Here's how the part is built. I have some questions about the finished solid (model axes, mm). Face numbers are marked on the shaded views. A direction names the side the tool comes from. Round coordinates to 2 decimals unless told otherwise and drop trailing zeros. Order: outer loops, then holes, each group sorted by start corner. A loop starts at its lowest first (then second) coordinate and runs counter-clockwise, first axis right, second up. Notation, with made-up numbers: (-26, -18) - (-13, -18) arc R13 cw to (-13, -10) - close; hole circle Ø7 at (-12, -30). An arc over 180 degrees is marked (long way). Answer as a JSON object with one key per item and string values.
```python
from build123d import *

# Parameters (mm, degrees)
SKETCH1_R               = 1.5
SKETCH1_R_2             = 3
SKETCH1_R_3             = 2
SKETCH1_W               = 12.75
SKETCH1_H               = 8.25
BOSS_EXTRUDE1_DEPTH     = 6.35
FILLET1_R               = 1.5
SKETCH3_W               = 129.678218063
SKETCH3_H               = 13.276015012
CUT_EXTRUDE1_DEPTH      = 56
SKETCH4_W               = 14.25
SKETCH4_H               = 6.35
SKETCH4_W_2             = 20.25
SKETCH4_W_3             = 16.5
BOSS_EXTRUDE2_DEPTH     = 25
SKETCH5_W               = 158.83803675
SKETCH5_H               = 69.224935419
CUT_EXTRUDE2_DEPTH      = 86
CUT_EXTRUDE3_DEPTH      = 10
CUT_EXTRUDE3_DEPTH_BACK = 49
SKETCH6_W               = 0.1
SKETCH6_H               = 6.35
SKETCH7_W               = 88.464513538
SKETCH7_H               = 23.115624737
CUT_EXTRUDE4_DEPTH      = 84


with BuildPart() as part:
    # Sketch1 → Boss-Extrude1 (new body)
    with BuildSketch(Plane(origin=(0, 0, 0), x_dir=(1, 0, 0), z_dir=(0, 1, 0))):
        Polygon((0, 20), (0, 104), (12, 104), (14, 93), (26, 93), (26, 107), (33.5, 114), (62.5, 114), (70, 107), (70, 93), (82, 93), (84, 104), (96, 104), (96, 20), (89, 9), (89, 0), (62, 0), (62, 8), (34, 8), (34, 0), (7, 0), (7, 9), align=None)
        with Locations(Location((12.5, 3, 0), (0, 0, 270))):
            Circle(SKETCH1_R, mode=Mode.SUBTRACT)
        with Locations(Location((28, 3, 0), (0, 0, 270))):
            Circle(SKETCH1_R, mode=Mode.SUBTRACT)
        with Locations(Location((68, 3, 0), (0, 0, 90))):
            Circle(SKETCH1_R, mode=Mode.SUBTRACT)
        with Locations(Location((83.5, 3, 0), (0, 0, 90))):
            Circle(SKETCH1_R, mode=Mode.SUBTRACT)
        with Locations(Location((14, 13, 0), (0, 0, 270))):
            Circle(SKETCH1_R_2, mode=Mode.SUBTRACT)
        with Locations(Location((27, 13, 0), (0, 0, 270))):
            Circle(SKETCH1_R_2, mode=Mode.SUBTRACT)
        with Locations(Location((69, 13, 0), (0, 0, 90))):
            Circle(SKETCH1_R_2, mode=Mode.SUBTRACT)
        with Locations(Location((82, 13, 0), (0, 0, 90))):
            Circle(SKETCH1_R_2, mode=Mode.SUBTRACT)
        with Locations(Location((22.75, 42.455027657, 0), (0, 0, 270))):
            Circle(SKETCH1_R, mode=Mode.SUBTRACT)
        with Locations(Location((22.75, 51.751081058, 0), (0, 0, 270))):
            Circle(SKETCH1_R, mode=Mode.SUBTRACT)
        with Locations(Location((73.25, 42.455027657, 0), (0, 0, 90))):
            Circle(SKETCH1_R, mode=Mode.SUBTRACT)
        with Locations(Location((73.25, 51.751081058, 0), (0, 0, 90))):
            Circle(SKETCH1_R, mode=Mode.SUBTRACT)
        with Locations(Location((18, 72.75, 0), (0, 0, 270))):
            Circle(SKETCH1_R, mode=Mode.SUBTRACT)
        with Locations(Location((28, 65.75, 0), (0, 0, 270))):
            Circle(SKETCH1_R, mode=Mode.SUBTRACT)
        with Locations(Location((68, 65.75, 0), (0, 0, 90))):
            Circle(SKETCH1_R, mode=Mode.SUBTRACT)
        with Locations(Location((78, 72.75, 0), (0, 0, 90))):
            Circle(SKETCH1_R, mode=Mode.SUBTRACT)
        with Locations(Location((36.5, 76.75, 0), (0, 0, 270))):
            Circle(SKETCH1_R_3, mode=Mode.SUBTRACT)
        with Locations(Location((59.5, 76.75, 0), (0, 0, 90))):
            Circle(SKETCH1_R_3, mode=Mode.SUBTRACT)
        with Locations(Location((35.5, 89, 0), (0, 0, 270))):
            Circle(SKETCH1_R, mode=Mode.SUBTRACT)
        with Locations(Location((35.5, 106.5, 0), (0, 0, 270))):
            Circle(SKETCH1_R, mode=Mode.SUBTRACT)
        with Locations(Location((60.5, 89, 0), (0, 0, 90))):
            Circle(SKETCH1_R, mode=Mode.SUBTRACT)
        with Locations(Location((60.5, 106.5, 0), (0, 0, 90))):
            Circle(SKETCH1_R, mode=Mode.SUBTRACT)
        with Locations(Location((44, 26, 0), (0, 0, 270))):
            Circle(SKETCH1_R, mode=Mode.SUBTRACT)
        with Locations(Location((52, 26, 0), (0, 0, 90))):
            Circle(SKETCH1_R, mode=Mode.SUBTRACT)
        with Locations(Location((52, 74, 0), (0, 0, 270))):
            Circle(SKETCH1_R, mode=Mode.SUBTRACT)
        with Locations(Location((44, 74, 0), (0, 0, 90))):
            Circle(SKETCH1_R, mode=Mode.SUBTRACT)
        with Locations(Location((48, 97.75, 0), (0, 0, 270))):
            Circle(SKETCH1_R_3, mode=Mode.SUBTRACT)
        with Locations((69.875, 25.875)):
            Rectangle(SKETCH1_W, SKETCH1_H, mode=Mode.SUBTRACT)
        with Locations((26.125, 25.875)):
            Rectangle(SKETCH1_W, SKETCH1_H, mode=Mode.SUBTRACT)
        with Locations((69.875, 81.875)):
            Rectangle(SKETCH1_W, SKETCH1_H, mode=Mode.SUBTRACT)
        with Locations((26.125, 81.875)):
            Rectangle(SKETCH1_W, SKETCH1_H, mode=Mode.SUBTRACT)
        with BuildLine():
            Line((3, 75), (7, 75))
            ThreePointArc((7, 75), (9, 73), (7, 71))
            Line((7, 71), (3, 71))
            ThreePointArc((3, 71), (1, 73), (3, 75))
        make_face(mode=Mode.SUBTRACT)
        with BuildLine():
            Line((93, 75), (89, 75))
            ThreePointArc((89, 75), (87, 73), (89, 71))
            Line((89, 71), (93, 71))
            ThreePointArc((93, 71), (95, 73), (93, 75))
        make_face(mode=Mode.SUBTRACT)
        with BuildLine():
            Line((93, 37), (89, 37))
            ThreePointArc((89, 37), (87, 35), (89, 33))
            Line((89, 33), (93, 33))
            ThreePointArc((93, 33), (95, 35), (93, 37))
        make_face(mode=Mode.SUBTRACT)
        with BuildLine():
            Line((3, 33), (7, 33))
            ThreePointArc((7, 33), (9, 35), (7, 37))
            Line((7, 37), (3, 37))
            ThreePointArc((3, 37), (1, 35), (3, 33))
        make_face(mode=Mode.SUBTRACT)
        with BuildLine():
            Line((15, 48.525154469), (23, 48.525154469))
            ThreePointArc((23, 48.525154469), (24.5, 47.025154469), (23, 45.525154469))
            Line((23, 45.525154469), (15, 45.525154469))
            ThreePointArc((15, 45.525154469), (13.5, 47.025154469), (15, 48.525154469))
        make_face(mode=Mode.SUBTRACT)
        with BuildLine():
            Line((81, 48.525154469), (73, 48.525154469))
            ThreePointArc((73, 48.525154469), (71.5, 47.025154469), (73, 45.525154469))
            Line((73, 45.525154469), (81, 45.525154469))
            ThreePointArc((81, 45.525154469), (82.5, 47.025154469), (81, 48.525154469))
        make_face(mode=Mode.SUBTRACT)
        with BuildLine():
            Line((16.5, 67.75), (16.5, 57.75))
            ThreePointArc((16.5, 57.75), (18, 56.25), (19.5, 57.75))
            Line((19.5, 57.75), (19.5, 67.75))
            ThreePointArc((19.5, 67.75), (18, 69.25), (16.5, 67.75))
        make_face(mode=Mode.SUBTRACT)
        with BuildLine():
            Line((76.5, 67.75), (76.5, 57.75))
            ThreePointArc((76.5, 57.75), (78, 56.25), (79.5, 57.75))
            Line((79.5, 57.75), (79.5, 67.75))
            ThreePointArc((79.5, 67.75), (78, 69.25), (76.5, 67.75))
        make_face(mode=Mode.SUBTRACT)
        with BuildLine():
            Line((46.5, 29), (38, 29))
            Line((38, 29), (38, 71))
            Line((38, 71), (46.5, 71))
            Line((46.5, 71), (46.5, 74))
            ThreePointArc((46.5, 74), (48, 75.5), (49.5, 74))
            Line((49.5, 74), (49.5, 71))
            Line((49.5, 71), (58, 71))
            Line((58, 71), (58, 29))
            Line((58, 29), (49.5, 29))
            Line((49.5, 29), (49.5, 26))
            ThreePointArc((49.5, 26), (48, 24.5), (46.5, 26))
            Line((46.5, 26), (46.5, 29))
        make_face(mode=Mode.SUBTRACT)
    extrude(amount=BOSS_EXTRUDE1_DEPTH)

    # Fillet1
    fillet1_edges = [part.edges().sort_by_distance(p)[0] for p in [
        (19.75, 3.175, -30),
        (19.75, 3.175, -21.75),
        (32.5, 3.175, -21.75),
        (32.5, 3.175, -30),
        (63.5, 3.175, -77.75),
        (76.25, 3.175, -77.75),
        (76.25, 3.175, -86),
        (63.5, 3.175, -86),
        (19.75, 3.175, -86),
        (19.75, 3.175, -77.75),
        (32.5, 3.175, -77.75),
        (32.5, 3.175, -86),
        (58, 3.175, -29),
        (58, 3.175, -71),
        (38, 3.175, -71),
        (38, 3.175, -29),
        (62, 3.175, -8),
        (34, 3.175, -8),
        (34, 3.175, 0),
        (7, 3.175, 0),
        (7, 3.175, -9),
        (0, 3.175, -20),
        (0, 3.175, -104),
        (12, 3.175, -104),
        (14, 3.175, -93),
        (26, 3.175, -93),
        (26, 3.175, -107),
        (33.5, 3.175, -114),
        (62.5, 3.175, -114),
        (70, 3.175, -107),
        (70, 3.175, -93),
        (82, 3.175, -93),
        (84, 3.175, -104),
        (96, 3.175, -104),
        (96, 3.175, -20),
        (89, 3.175, -9),
        (89, 3.175, 0),
        (62, 3.175, 0),
        (76.25, 3.175, -21.75),
        (76.25, 3.175, -30),
        (63.5, 3.175, -30),
        (63.5, 3.175, -21.75),
    ]]
    fillet(fillet1_edges, radius=FILLET1_R)

    # Sketch3 → Cut-Extrude1 (cut)
    with BuildSketch(Plane(origin=(48, 0, 0), x_dir=(0, 0, -1), z_dir=(1, 0, 0))):
        with Locations((58.42243018, 0.940732076)):
            Rectangle(SKETCH3_W, SKETCH3_H)
    extrude(amount=CUT_EXTRUDE1_DEPTH, mode=Mode.SUBTRACT)

    # Sketch4 → Boss-Extrude2 (add)
    with BuildSketch(Plane(origin=(48, 0, 0), x_dir=(0, 0, -1), z_dir=(1, 0, 0))):
        with Locations((106.875, 3.175)):
            Rectangle(SKETCH4_W, SKETCH4_H)
        with Locations((85.625, 3.175)):
            Rectangle(SKETCH4_W_2, SKETCH4_H)
        with Locations((16.25, 3.175)):
            Rectangle(SKETCH4_W_3, SKETCH4_H)
    extrude(amount=BOSS_EXTRUDE2_DEPTH)

    # Mirror1: part across plane


with BuildPart() as part_1:
    add(part.part)
    add(part.part.mirror(Plane(origin=(73, 0, 0), x_dir=(0, 0, 1), z_dir=(1, 0, 0))))

    # Sketch5 → Cut-Extrude2 (cut)
    with BuildSketch(Plane(origin=(75, 0, 0), x_dir=(0, 0, -1), z_dir=(1, 0, 0))):
        with Locations((54.73207584, 3.767679241)):
            Rectangle(SKETCH5_W, SKETCH5_H)
    extrude(amount=CUT_EXTRUDE2_DEPTH, mode=Mode.SUBTRACT)

    # Sketch6 → Cut-Extrude3 (cut, two sides: drawn at the far end of the back side and taken through both)
    with BuildSketch(Plane(origin=(38, 0, 0), x_dir=(0, 0, -1), z_dir=(1, 0, 0)).offset(-CUT_EXTRUDE3_DEPTH_BACK)):
        with Locations((48.95, 3.175)):
            Rectangle(SKETCH6_W, SKETCH6_H)
    extrude(amount=CUT_EXTRUDE3_DEPTH + CUT_EXTRUDE3_DEPTH_BACK, mode=Mode.SUBTRACT)


with BuildPart() as cut_extrude3_piece_1:
    # of the separate pieces the step leaves, piece 1, a body of its own (cut_extrude3_pieces)
    add(part_1.part.solids().sort_by_distance((0, 0, -49))[0])

    # Sketch7 → Cut-Extrude4 (cut)
    with BuildSketch(Plane(origin=(0, 0, -48.91), x_dir=(-1, 0, 0), z_dir=(0, 0, -1))):
        with Locations((-38.621683349, 5.173992705)):
            Rectangle(SKETCH7_W, SKETCH7_H)
    extrude(amount=CUT_EXTRUDE4_DEPTH, mode=Mode.SUBTRACT)


with BuildPart() as cut_extrude3_piece_2:
    # of the separate pieces the step leaves, piece 2, a body of its own (cut_extrude3_pieces)
    add(part_1.part.solids().sort_by_distance((0, 0, -20.436801031))[0])


solid = cut_extrude3_piece_2.part
```
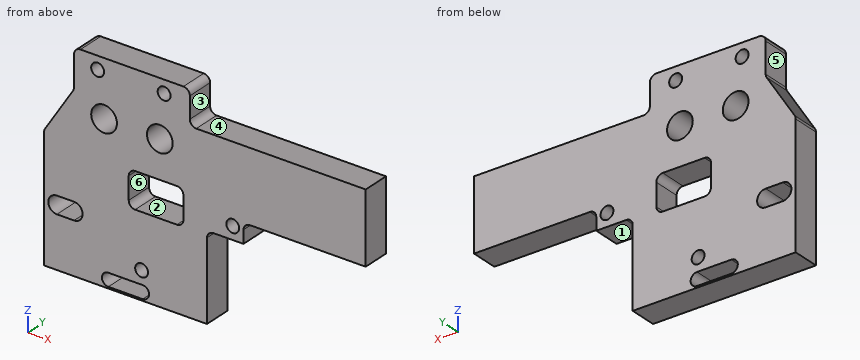
1. Imagine slicing it at D-D (x = 12.5). List the corners of the cut face in (y, z) for me.
Responses:
{"outline": "(0, -48.9) - (6.35, -48.9) - (6.35, -15.6) - (0, -15.6) - close; (0, -10.4) - (6.35, -10.4) - (6.35, -4.5) - (0, -4.5) - close; (0, -1.5) - (6.35, -1.5) - (6.35, 0) - (0, 0) - close"}
2. For the marked faces 1, 2 and 3, which set-ups out of +Z, -Z, +X, -X, +Y, -Y let a thin tool reach every point of the face, with its end or its side?
Responses:
{"face 1": "-Z, +X, +Y, -Y", "face 2": "+Y, -Y", "face 3": "+Z, +X, +Y, -Y"}
3. If I drill on L1, parallel to X at y = 3.5, z = -3; L2, parallel to X at y = 3.75, z = -26; L3, parallel to Z at x = 16.5, y = 2, over which ranges is the centre line in solid material (lowest first)? Write a range as [from, to].
Responses:
{"L1": "[7, 11], [14, 26.5], [29.5, 34]", "L2": "[0, 19.75], [32.5, 42.5], [45.5, 46.5]", "L3": "[-48.9, -48.53], [-45.53, -14.66], [-11.34, 0]"}
4. Imagine slicing it at A-A (z = -11). List the corners of the cut face in (x, y) for me, plus the area to 3 significant figures.
Responses:
{"outline": "(5.73, 0) - (11.76, 0) - (11.76, 6.35) - (5.73, 6.35) - close; (16.24, 0) - (24.76, 0) - (24.76, 6.35) - (16.24, 6.35) - close; (29.24, 0) - (75, 0) - (75, 6.35) - (29.24, 6.35) - close", "area": "383 mm2"}
5. Imagine slicing it at B-B (y = 4.5). Give the number of separate pieces and of enclosed holes in the cut face, plus the area to 3 significant figures.
Responses:
{"separate pieces": "1", "enclosed holes": "9", "area": "2,130 mm2"}
6. For P1, Ø8, axis at x = 27, z = -13, coming from the -Y side; P2, Ø2, axis at x = 4.5, y = 2.5, coming from the +Z side; P3, Ø1.8, axis at x = 44, z = -26, coming from the -Y side; P4, Ø1.9, axis at x = 41.5, y = 4, coming from the -Z side, each with a flat end and sliding along its axis, tell me the tip position at first contact or that it passes through.
Responses:
{"P1": "y = 0", "P2": "z = -11.36", "P3": "through", "P4": "z = -29"}
7. Imagine slicing it at C-C (x = 28). List the corners of the cut face in (y, z) for me, plus the area to 3 significant figures.
Responses:
{"outline": "(0, -48.9) - (6.35, -48.9) - (6.35, -30) - (0, -30) - close; (0, -21.75) - (6.35, -21.75) - (6.35, -15.83) - (0, -15.83) - close; (0, -10.17) - (6.35, -10.17) - (6.35, -4.5) - (0, -4.5) - close; (0, -1.5) - (6.35, -1.5) - (6.35, 0) - (0, 0) - close", "area": "203 mm2"}
8. Thinking about a two-plate mould opening in Z: for the marked faces 4, 5 and 6, which applies, pulls with the +Z half, pulls with the -Z half, needs draft (parallel to the pull), parting line crosses it, or undercut?
Responses:
{"face 4": "pulls with the +Z half", "face 5": "needs draft", "face 6": "undercut"}
